Can you work these out from the model? Positions are in its coordinate system, mm. A direction names the side the tool comes from. Round coordinates to 2 decimals unless told otherwise and drop trailing zeros. Write each loop counter-clockwise with the first axis right and the second up, starting at its lowest first coordinate (ties: lowest second). Pieces come first, ordered by that corner, then holes.
Q1. If we section it at A-A (y = -49.5): Please give me the cut outline in (x, z).
Q2. If we section it at B-B (x = -1): Please give me the cut outline in (y, z), plus the area to 3 significant figures.
Q3. Please list where these lines run through material, in increasing order: line 1 along Z through (x, y) = (11.25, -49.5); line 2 along X through (y, z) = (111, 7.5); line 3 along Z through (x, y) = (12.5, 13).
Q4. For faces 1 (the flat face through (-10, -10, -12)), 2 (the cylindrical face through (-14.014, 118.747, 0.247)), 3 (the cylindrical face through (-12.5, 112.5, -0.1)), 4 (the flat face through (0, -2, 11.25)), which set-ups out of +Z, -Z, +X, -X, +Y, -Y let a thin tool reach every point of the face, with its end or its side?
Q5. We'd pull the mould along X, two halves only. Please class faces 5 (the flat face through (15, -1.8, 11.4)), 6 (the flat face through (10, -1, -13)), 7 (the flat face through (-13, 1.7, 5.2)): +X half, -X half, draft (parallel to the pull), parting line (faces both ways), or undercut.
Q6. I'm going to push flat-ended pins straight in: pin 1 Ø12 at (x, z) = (7.5, -4) entering from -Y; pin 2 Ø7 at (y, z) = (20.5, -4) entering from +X; pin 3 Ø1.5 at (x, y) = (-7.5, -73.5) entering from -Z; pin 4 Ø5 at (x, z) = (10, 6.5) entering from -Y. Where does each tip first touch, or does it pass through?
from build123d import *

# Parameters (mm, degrees)
F1_DEPTH      = 125
F1_DEPTH_BACK = 125
F6_DEPTH      = 5.001
F7_DEPTH      = 5.001
F8_DEPTH      = 2
F9_DEPTH      = 2
F10_DEPTH     = 2
F11_DEPTH     = 2
F12_T1_DEPTH  = 92.5
F12_T3_DEPTH  = 92.5
F12_T5_DEPTH  = 117.5


# Not quite as in the source:
# - a fillet or chamfer that OpenCascade refuses, or shapes differently, is made with other operations: its cross-section is extruded or revolved along the edge and cut away or added


with BuildPart() as f1:
    # F0 (on Front) → F1 (new body, two sides)
    with BuildSketch(Plane.XZ) as f1_sk:
        Polygon((15, -17.5), (15, 17.5), (-15, 17.5), (-15, -17.5), (-10, -17.5), (-10, 11.25), (10, 11.25), (10, -17.5), align=None)
    extrude(amount=F1_DEPTH)
    extrude(f1_sk.sketch, amount=-F1_DEPTH_BACK)

    # F2 (on face) → F6 (cut, through all)
    with BuildSketch(Plane(origin=(10, 0, 0), x_dir=(0, -1, 0), z_dir=(-1, 0, 0))):
        with BuildLine():
            Line((-107.5, -5), (107.5, -5))
            ThreePointArc((107.5, -5), (112.5, 0), (107.5, 5))
            Line((107.5, 5), (-107.5, 5))
            ThreePointArc((-107.5, 5), (-112.5, 0), (-107.5, -5))
        make_face()
    extrude(amount=-F6_DEPTH, mode=Mode.SUBTRACT)

    # F4 (on face) → F7 (cut, through all)
    with BuildSketch(Plane.YZ.offset(-10)):
        with BuildLine():
            Line((107.5, 5), (-107.5, 5))
            ThreePointArc((-107.5, 5), (-112.5, 0), (-107.5, -5))
            Line((-107.5, -5), (107.5, -5))
            ThreePointArc((107.5, -5), (112.5, 0), (107.5, 5))
        make_face()
    extrude(amount=-F7_DEPTH, mode=Mode.SUBTRACT)

    # F2 (on face) → F8 (cut)
    with BuildSketch(Plane(origin=(10, 0, 0), x_dir=(0, -1, 0), z_dir=(-1, 0, 0))):
        with BuildLine():
            Line((-107.5, -11.25), (107.5, -11.25))
            ThreePointArc((107.5, -11.25), (118.75, 0), (107.5, 11.25))
            Line((107.5, 11.25), (-107.5, 11.25))
            ThreePointArc((-107.5, 11.25), (-118.75, 0), (-107.5, -11.25))
        make_face()
        with BuildLine():
            ThreePointArc((107.5, 5), (112.5, 0), (107.5, -5))
            Line((107.5, -5), (-107.5, -5))
            ThreePointArc((-107.5, -5), (-112.5, 0), (-107.5, 5))
            Line((-107.5, 5), (107.5, 5))
        make_face(mode=Mode.SUBTRACT)
    extrude(amount=-F8_DEPTH, mode=Mode.SUBTRACT)

    # F3 (on face) → F9 (cut)
    with BuildSketch(Plane.YZ.offset(15)):
        with BuildLine():
            ThreePointArc((-107.5, 11.25), (-118.75, 0), (-107.5, -11.25))
            Line((-107.5, -11.25), (107.5, -11.25))
            ThreePointArc((107.5, -11.25), (118.75, 0), (107.5, 11.25))
            Line((107.5, 11.25), (-107.5, 11.25))
        make_face()
        with BuildLine():
            ThreePointArc((-107.5, -5), (-112.5, 0), (-107.5, 5))
            Line((-107.5, 5), (107.5, 5))
            ThreePointArc((107.5, 5), (112.5, 0), (107.5, -5))
            Line((107.5, -5), (-107.5, -5))
        make_face(mode=Mode.SUBTRACT)
    extrude(amount=-F9_DEPTH, mode=Mode.SUBTRACT)

    # F5 (on face) → F10 (cut)
    with BuildSketch(Plane(origin=(-15, 0, 0), x_dir=(0, -1, 0), z_dir=(-1, 0, 0))):
        with BuildLine():
            Line((107.5, 11.25), (-107.5, 11.25))
            ThreePointArc((-107.5, 11.25), (-118.75, 0), (-107.5, -11.25))
            Line((-107.5, -11.25), (107.5, -11.25))
            ThreePointArc((107.5, -11.25), (118.75, 0), (107.5, 11.25))
        make_face()
        with BuildLine():
            ThreePointArc((-107.5, -5), (-112.5, 0), (-107.5, 5))
            Line((-107.5, 5), (107.5, 5))
            ThreePointArc((107.5, 5), (112.5, 0), (107.5, -5))
            Line((107.5, -5), (-107.5, -5))
        make_face(mode=Mode.SUBTRACT)
    extrude(amount=-F10_DEPTH, mode=Mode.SUBTRACT)

    # F4 (on face) → F11 (cut)
    with BuildSketch(Plane.YZ.offset(-10)):
        with BuildLine():
            Line((107.5, 11.25), (-107.5, 11.25))
            ThreePointArc((-107.5, 11.25), (-118.75, 0), (-107.5, -11.25))
            Line((-107.5, -11.25), (107.5, -11.25))
            ThreePointArc((107.5, -11.25), (118.75, 0), (107.5, 11.25))
        make_face()
        with BuildLine():
            ThreePointArc((-107.5, -5), (-112.5, 0), (-107.5, 5))
            Line((-107.5, 5), (107.5, 5))
            ThreePointArc((107.5, 5), (112.5, 0), (107.5, -5))
            Line((107.5, -5), (-107.5, -5))
        make_face(mode=Mode.SUBTRACT)
    extrude(amount=-F11_DEPTH, mode=Mode.SUBTRACT)

    # F12: fillet of radius 17.5 on 6 edges, made by hand

    # F12_s2 → F12_t1 (cut)
    with BuildSketch(Plane.YZ.offset(-58.75)):
        with BuildLine():
            ThreePointArc((125, 0), (119.8743686708, -12.3743686708), (107.5, -17.5))
            Line((107.5, -17.5), (125, -17.5))
            Line((125, -17.5), (125, 0))
        make_face()
        with BuildLine():
            ThreePointArc((-125, 0), (-119.8743686708, -12.3743686708), (-107.5, -17.5))
            Line((-107.5, -17.5), (-125, -17.5))
            Line((-125, -17.5), (-125, 0))
        make_face()
    extrude(amount=F12_T1_DEPTH, mode=Mode.SUBTRACT)

    # F12_s4 → F12_t3 (cut)
    with BuildSketch(Plane.YZ.offset(-33.75)):
        with BuildLine():
            ThreePointArc((107.5, -17.5), (119.8743686708, -12.3743686708), (125, 0))
            Line((125, 0), (125, -17.5))
            Line((125, -17.5), (107.5, -17.5))
        make_face()
        with BuildLine():
            ThreePointArc((-107.5, -17.5), (-119.8743686708, -12.3743686708), (-125, 0))
            Line((-125, 0), (-125, -17.5))
            Line((-125, -17.5), (-107.5, -17.5))
        make_face()
    extrude(amount=F12_T3_DEPTH, mode=Mode.SUBTRACT)

    # F12_s6 → F12_t5 (cut)
    with BuildSketch(Plane.YZ.offset(-58.75)):
        with BuildLine():
            ThreePointArc((125, 0), (119.8743686708, 12.3743686708), (107.5, 17.5))
            Line((107.5, 17.5), (125, 17.5))
            Line((125, 17.5), (125, 0))
        make_face()
        with BuildLine():
            ThreePointArc((-125, 0), (-119.8743686708, 12.3743686708), (-107.5, 17.5))
            Line((-107.5, 17.5), (-125, 17.5))
            Line((-125, 17.5), (-125, 0))
        make_face()
    extrude(amount=F12_T5_DEPTH, mode=Mode.SUBTRACT)


solid = f1.part
A:
1. outline: (-15, -17.5) - (-10, -17.5) - (-10, -11.25) - (-12, -11.25) - (-12, -5) - (-13, -5) - (-13, -11.25) - (-15, -11.25) - close; (-15, 11.25) - (-13, 11.25) - (-13, 5) - (-12, 5) - (-12, 11.25) - (12, 11.25) - (12, 5) - (13, 5) - (13, 11.25) - (15, 11.25) - (15, 17.5) - (-15, 17.5) - close; (10, -17.5) - (15, -17.5) - (15, -11.25) - (13, -11.25) - (13, -5) - (12, -5) - (12, -11.25) - (10, -11.25) - close
2. outline: (-120.9, 11.25) - (120.9, 11.25) arc R17.5 ccw to (107.5, 17.5) - (-107.5, 17.5) arc R17.5 ccw to start
2. area: 1,460 mm2
3. line 1: z = -17.5 to -11.25, 11.25 to 17.5
3. line 2: x = -13 to -12, 12 to 13
3. line 3: z = -17.5 to -5, 5 to 17.5
4. face 1: -Z, +Y, -Y
4. face 2: -X
4. face 3: +X, -X
4. face 4: none
5. face 5: +X half
5. face 6: undercut
5. face 7: -X half
6. pin 1: stops at y = -125
6. pin 2: stops at x = 13
6. pin 3: stops at z = 11.25
6. pin 4: stops at y = -124.54
